Check sheet for the drawn part. Datum: minimum x, y, z corner. Units: mm. A direction names the side the tool comes from. Give positions to 0.01 mm unless a question says otherwise; leave off trailing zeros. Order: outer loops, then holes, each group sorted by start corner. A loop starts at its lowest first (then second) coordinate and runs counter-clockwise, first axis right, second up. Notation, with made-up numbers: M 41,32.25 L 64,32.25 A13 cw 64,38.25 Z; hole C 2.5,1.5 d8. An arc over 180 degrees is marked long. Put each result on its own line as item: value. Start each with the question number.
Q1. Section check C-C on y = 3.8. Record the cut outline in (x, z), then the cut area to 3 significant figures.
Q2. Section check B-B on x = 3.75. Record the cut outline in (y, z), then the cut area to 3 significant figures.
Q3. Material ranges on L1, parallel to Y at x = 7.25, z = 2.5; L2, parallel to Z at x = 22.5, y = 4.9; L3, parallel to Z at x = 7, y = 5.1, recorded low to high.
Q4. Go/stop test with a flat-tipped pin: pin 1 (1.5 mm diameter, centred on x = 18, y = 3, fed in from +Z). Record where the tip stops, or that it passes through.
Q5. Section check A-A on z = 4.1. Record the cut outline in (x, y).
Q6. Access from +Z, -Z, +X, -X, +Y, -Y to the whole of each face (thin tool, end or side, straight path). Record for the marked faces 1 and 2.
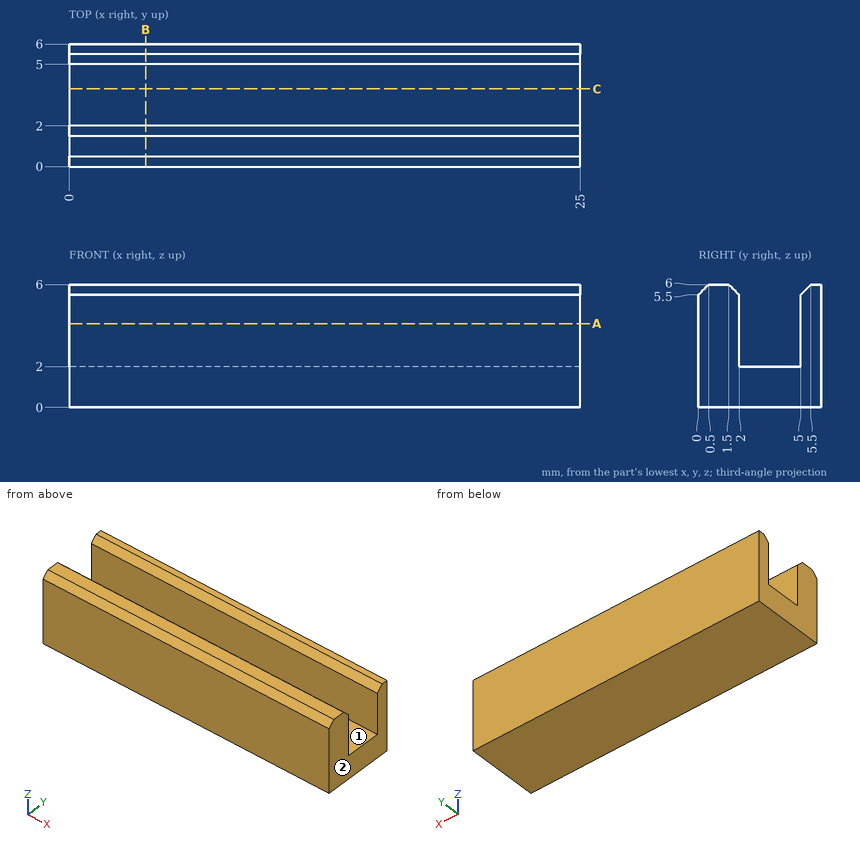
Results found:
1. outline: M 0,0 L 25,0 L 25,2 L 0,2 Z
1. area: 50.0 mm^2
2. outline: M 0,0 L 6,0 L 6,6 L 5.5,6 L 5,5.5 L 5,2 L 2,2 L 2,5.5 L 1.5,6 L 0.5,6 L 0,5.5 Z
2. area: 23.6 mm^2
3. L1: y = 0 to 2, 5 to 6
3. L2: z = 0 to 2
3. L3: z = 0 to 5.6
4. pin 1: stops at z = 2
5. outline: M 0,0 L 25,0 L 25,2 L 0,2 Z; M 0,5 L 25,5 L 25,6 L 0,6 Z
6. face 1: +Z, +X, -X
6. face 2: +Z, -Z, +X, +Y, -Y
